Autodesk Inventor part; units mm, degrees
ref_plane "YZ Plane" through (0, 0, 0) normal (1, 0, 0) x (0, 1, 0)
ref_plane "XZ Plane" through (0, 0, 0) normal (0, 1, 0) x (-1, 0, 0)
ref_plane "XY Plane" through (0, 0, 0) normal (0, 0, 1) x (1, 0, 0)
sketch "草图1" plane through (0, 0, 0) normal (0, 0, 1) x (1, 0, 0)
  line L0 (140, -71) -> (-140, -71)
  line L1 (-140, -71) -> (-140, 71)
  line L2 (-140, 71) -> (140, 71)
  line L3 (140, 71) -> (140, -71)
  line L4 (140, -71) -> (-140, 71) construction
  line L5 (-140, -71) -> (140, 71) construction
  point P0 (0, 0)
  dimension "d0" = 280
  dimension "d1" = 142
extrude "拉伸1" add sketch "草图1" along normal blind 5
sketch "草图2" plane through (0, 0, 5) normal (0, 0, 1) x (1, 0, 0)
  line L0 (110, 27.873) -> (110, -28.2358)
  line L1 (-140, -71) -> (140, -71)
  line L2 (0, -71) -> (0, 71)
  line L3 (140, 71) -> (-140, 71)
  circle A0 centre (0, 0) radius 24.4986
sketch "草图3" plane through (0, 0, 5) normal (0, 0, 1) x (1, 0, 0)
  point P0 (0, 0)
sketch "草图4" plane through (0, 0, 5) normal (0, 0, 1) x (1, 0, 0)
  circle A0 centre (117, 63.8186) radius 1.85
  circle A1 centre (133, 63.8186) radius 1.85
  circle A2 centre (117, -64.1814) radius 1.85
  circle A3 centre (133, -64.1814) radius 1.85
  line L0 (140, -32.9821) -> (110, -32.9821)
  line L1 (110, 32.6193) -> (140, 32.6193)
  line L2 (140, -71) -> (140, 71)
  line L3 (140, -41.9821) -> (73.7163, -41.9821)
  line L4 (73.7163, -41.9821) -> (73.7163, 41.6193)
  line L5 (73.7163, 41.6193) -> (140, 41.6193)
  line L6 (140, 41.6193) -> (140, -41.9821)
  point P0 (0, 0)
  dimension "d4" = 9
  dimension "d5" = 9
extrude "拉伸2" cut sketch "草图4" against normal blind 5
ref_plane "工作平面1" through (0, 71, 5) normal (1, 0, 0) x (0, 0, -1)
mirror "镜像1" about plane through (0, 71, 5) normal (1, 0, 0) of "拉伸2"
fillet "圆角1" radius 5 4 edges at (73.7163, -41.9821, 2.5) (73.7163, 41.6193, 2.5) (-73.7163, 41.6193, 2.5) (-73.7163, -41.9821, 2.5)
extrude "拉伸3" cut sketch "草图2" against normal blind 10
properties part number "玻纤"
Part model, mm, in its own coordinate system. A direction names the side the tool comes from. Give positions to 0.01 mm unless a question says otherwise; leave off trailing zeros. Order: outer loops, then holes, each group sorted by start corner. A loop starts at its lowest first (then second) coordinate and runs counter-clockwise, first axis right, second up. Notation, with made-up numbers: (32, 18.25) - (58, 18.25) arc R29 cw to (58, 39.25) - close; hole circle Ø2 at (-19, 82.25). An arc over 180 degrees is marked (long way). One line per question, with ' | ' between items.
1. Pull direction X, two halves, no side cores. Call faces 1 (the face through (-109, -41.982, 3)), 2 (the face through (-73.716, 0, 3)), 3 (the face through (-18.056, 16.557, 2.535)), 4 (the face through (75.142, 40.116, 2.465)): +X half, -X half, draft (parallel to the pull), parting line (faces both ways), or undercut.
Filled in:
face 1: draft | face 2: -X half | face 3: undercut | face 4: +X half
2. Which spindle directions (+Z, -Z, +X, -X, +Y, -Y) get a long thin tool onto all of the face, cutting with end or side? Do faces 5 (the face through (-33, 1, 5)), 6 (the face through (73.716, -1, 3)), 7 (the face through (-110, 41.619, 3)). Say none if no direction does.
Filled in:
face 5: +Z, +X, -X, +Y, -Y | face 6: +Z, -Z, +X | face 7: +Z, -Z, -X
3. Band-saw the part on A-A on y = 0. List the corners of the cut face in (x, z).
Filled in:
outline: (-73.72, 0) - (-24.5, 0) - (-24.5, 5) - (-73.72, 5) - close; (24.5, 0) - (73.72, 0) - (73.72, 5) - (24.5, 5) - close
4. Band-saw the part on B-B on x = 0. List the corners of the cut face in (y, z).
Filled in:
outline: (-71, 0) - (-24.5, 0) - (-24.5, 5) - (-71, 5) - close; (24.5, 0) - (71, 0) - (71, 5) - (24.5, 5) - close
5. Drill centre lines: probe 1 along Y at (x, z) = (-117, 2.95); probe 2 along X at (y, z) = (1, 4.75); probe 3 along Y at (x, z) = (-78, 2.65). Where is each one in solid material? Low to high.
Filled in:
probe 1: -71 to -66.03, -62.33 to -41.98, 41.62 to 61.97, 65.67 to 71 | probe 2: -73.72 to -24.48, 24.48 to 73.72 | probe 3: -71 to -41.93, 41.57 to 71
6. Band-saw the part on C-C on z = 3.8. Give the number of separate pieces and of enclosed holes in the cut face, then the cut area to 3 significant figures.
Filled in:
separate pieces: 1 | enclosed holes: 9 | area: 26,700 mm²
7. Drop flat-ended pins along their axis: P1, Ø3.5, axis at x = 117, y = 63.82, coming from the +Z side; P2, Ø8, axis at x = -105.5, y = -46.5, coming from the -Z side; P3, Ø1.5, axis at y = 0, z = 2, coming from the -X side; P4, Ø2.5, axis at y = -7.5, z = 3.5, coming from the +X side. Give the stop position or say it passes through.
Filled in:
P1: through | P2: z = 0 | P3: x = -73.72 | P4: x = 73.72
